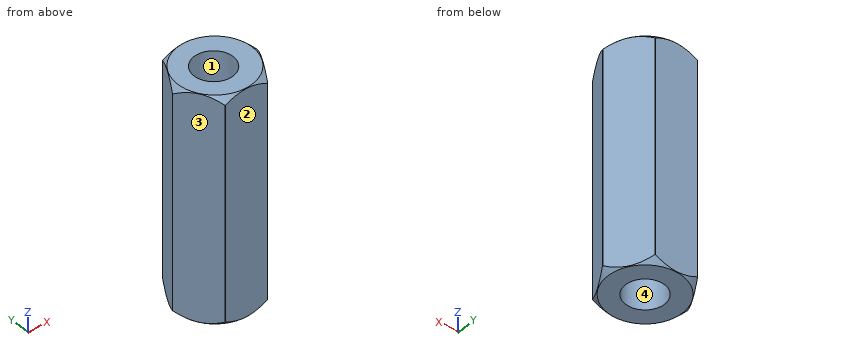
Autodesk Inventor part; units mm, degrees
ref_plane "Work Plane1" through (-1.711, 0.0003, 0) normal (0, 1, 0) x (1, 0, 0)
ref_plane "Work Plane2" through (0.1135, 0.0003, 9.525) normal (0, 0, -1) x (-1, 0, 0)
ref_plane "YZ Plane" through (0, 0, 0) normal (1, 0, 0) x (0, 1, 0)
sketch "Sketch1" plane through (0, 0, 0) normal (0, 0, 1) x (1, 0, 0)
  line L0 (1.9552, -3.1747) -> (-1.711, -3.1747)
  line L1 (-1.711, -3.1747) -> (-3.5441, 0.0003)
  line L2 (-3.5441, 0.0003) -> (-1.711, 3.1753)
  line L3 (-1.711, 3.1753) -> (1.9552, 3.1753)
  line L4 (1.9552, 3.1753) -> (3.7883, 0.0003)
  line L5 (3.7883, 0.0003) -> (1.9552, -3.1747)
  point P0 (0.1221, 0.0003)
  dimension "d0" = 6.35
extrude "Extrusion1" add sketch "Sketch1" along normal blind 19.05
ref_plane "Work Plane1" through (-1.711, 0.0003, 0) normal (0, 1, 0) x (1, 0, 0)
sketch "Sketch3" plane through (-1.711, 0.0003, 0) normal (0, 1, 0) x (1, 0, 0)
  line L0 (-1.3251, 0) -> (4.9741, 0)
  line L1 (5.4821, -0.508) -> (5.4821, -18.542)
  line L2 (-1.8331, -18.542) -> (-1.8331, -0.508)
  line L3 (-1.8331, -0.508) -> (-1.3251, 0)
  line L4 (4.9741, 0) -> (5.4821, -0.508)
  line L5 (-1.8331, 0) -> (-1.8331, -19.05)
  line L6 (3.6662, 0) -> (5.4993, 0)
  line L7 (1.8245, 0) -> (1.8245, -19.05)
  line L8 (0, -19.05) -> (-1.8331, -19.05)
  line L9 (5.4993, -19.05) -> (3.6662, -19.05)
  line L10 (3.6662, -19.05) -> (0, -19.05)
  line L11 (-1.3251, -19.05) -> (-1.8331, -18.542)
  line L12 (4.9741, -19.05) -> (5.4821, -18.542)
  point P0 (-1.8331, 0)
  point P1 (5.4821, 0)
  point P2 (5.4821, -19.05)
  dimension "d5" = 0.508
  dimension "d6" = 0.508
  dimension "d7" = 0.508
  dimension "d8" = 0.508
  dimension "d16" = 0
  dimension "d46" = 0.508
  dimension "d47" = 0.508
  dimension "d48" = 0.508
  dimension "d49" = 0.508
revolve "Revolution1" cut sketch "Sketch3" angle 360 about axis through (0.1135, 0.0003, 0) along (0, 0, 1) keep common part contours L0 L4 L1 L12 L9 L10 L7
sketch "Sketch6" plane through (0.1135, 0.0003, 0) normal (0, 0, -1) x (-1, 0, 0)
  circle A0 centre (0, 0) radius 3.1496
hole "Hole3" at (0.1135, 0.0003, 0) direction (0, 0, 1) diameter 3.302 depth 6.35 tip angle 118
sketch "Sketch7" plane through (0, 0, 19.05) normal (0, 0, 1) x (1, 0, 0)
  point P0 (0, 0)
hole "Hole4" at (0, 0, 19.05) direction (0, 0, -1) diameter 3.302 depth 6.35 tip angle 118
ref_plane "Work Plane2" through (0.1135, 0.0003, 9.525) normal (0, 0, -1) x (-1, 0, 0)
properties part number "0.75 inch Standoff" material "Steel"
Verification items for the finished model (mm, model axes). Face numbers are marked on the shaded views. Give positions to 0.01 mm unless a question says otherwise; leave off trailing zeros.
1. Go/stop test with flat-tipped pins: P1, Ø3, axis at y = -1, z = 15, coming from the -X side; P2, Ø2, axis at x = 0, y = 0, coming from the -Z side. Record where each tip stops, or that it passes through.
Derived:
P1: stops at x = -3.54
P2: stops at z = 6.67
2. Release check for a two-part mould opening along X. For the marked faces 1, 2, 3 and 4 record: +X half, -X half, draft (parallel to the pull), parting line (faces both ways), or undercut.
Derived:
face 1: undercut
face 2: draft
face 3: -X half
face 4: undercut
3. Material ranges on probe 1 along Y at (x, z) = (0, 17.5); probe 2 along Y at (x, z) = (0.5, 18); probe 3 along X at (y, z) = (-2, 2), recorded low to high.
Derived:
probe 1: y = -3.17 to -1.65, 1.65 to 3.18
probe 2: y = -3.17 to -1.57, 1.57 to 3.18
probe 3: x = -2.39 to 2.63
